Verification items for this drawing (mm, ordinates from the low corner). Give positions to 0.01 mm unless a question says otherwise; leave off trailing zeros. Order: outer loops, then holes, each group sorted by start corner. A loop starts at its lowest first (then second) coordinate and runs counter-clockwise, first axis right, second up. Notation, with made-up numbers: (58.25, 6) - (105.25, 6) arc R30 cw to (105.25, 35) - close; hole circle Ø1 at (-25, 63). An arc over 180 degrees is marked (long way). Put each result on its own line as item: value. Start each with the question number.
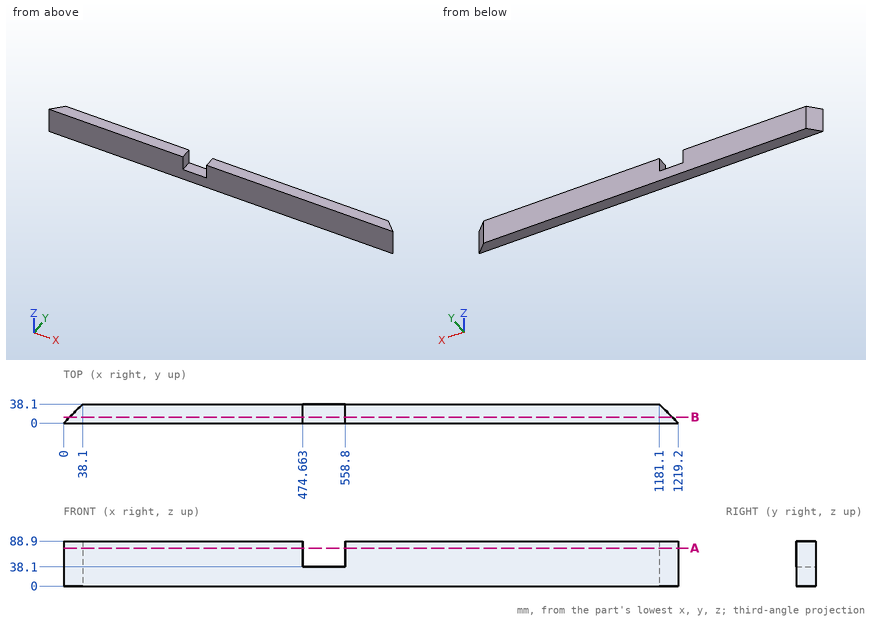
Item 1: Cross-section at A-A (z = 75). Enter the section's corners in (x, y), and give its area (3 significant figures).
Item 2: Thickness scan on line 1 along X through (y, z) = (11, 71) (1 decimal); line 2 along X through (y, z) = (9, 66) (1 decimal); line 3 along X through (y, z) = (32, 19). Record the ranges inside material, lowest first.
Item 3: Gauge pin test, flat ends, axial feed: pin 1 Ø11.5 at (y, z) = (13, 61) entering from +X; pin 2 Ø1 at (y, z) = (24, 43.5) entering from +X; pin 3 Ø3 at (y, z) = (13.5, 41.5) entering from -X. Record the tip position at first contact, or that the pin passes through.
Item 4: Cross-section at B-B (y = 12). Enter the section's corners in (x, z).
Recorded:
1. outline: (0, 0) - (474.66, 0) - (474.66, 38.1) - (38.1, 38.1) - close; (558.8, 0) - (1219.2, 0) - (1181.1, 38.1) - (558.8, 38.1) - close
1. area: 41,800 mm^2
2. line 1: x = 11 to 474.7, 558.8 to 1208.2
2. line 2: x = 9 to 474.7, 558.8 to 1210.2
2. line 3: x = 32 to 1187.2
3. pin 1: stops at x = 1211.95
3. pin 2: stops at x = 1195.7
3. pin 3: stops at x = 12
4. outline: (12, 0) - (1207.2, 0) - (1207.2, 88.9) - (558.8, 88.9) - (558.8, 38.1) - (474.66, 38.1) - (474.66, 88.9) - (12, 88.9) - close
